The figure shows three views and two pictorial views of one solid part (mm, origin at its lowest corner). Answer the questions. Round coordinates to 2 decimals unless told otherwise and drop trailing zeros. Order: outer loops, then holes, each group sorted by start corner. A loop starts at its lowest first (then second) coordinate and runs counter-clockwise, first axis right, second up. Notation, with made-up numbers: M 4.5,58 L 35.5,58 A15 cw 35.5,75 Z; hole C -29,2.25 d10. An arc over 180 degrees is marked long. Return JSON: item names as keys, results as strings.
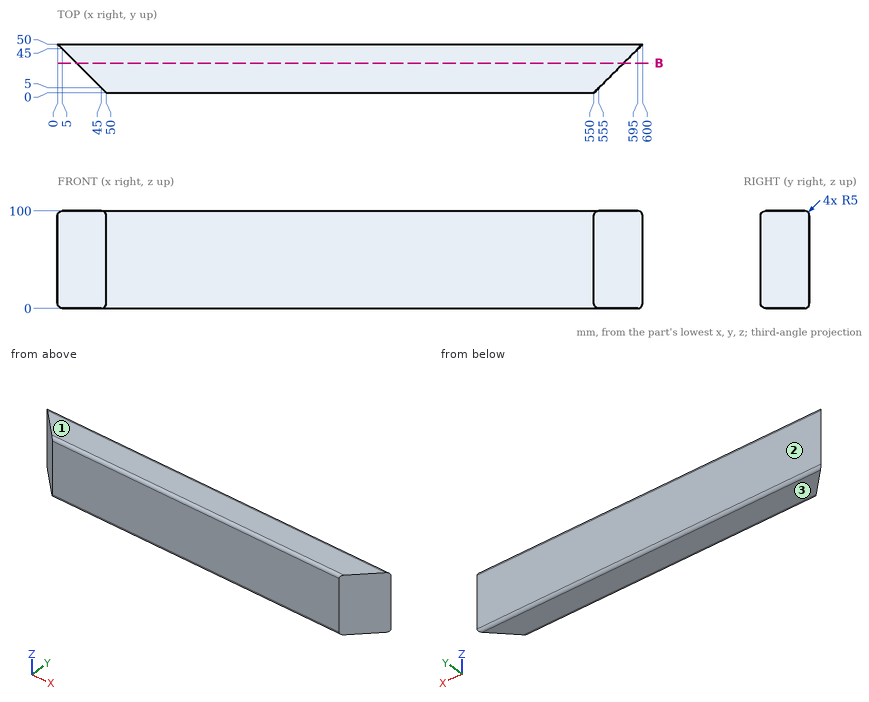
Item 1: Each of these flat-tipped pins is pushed along its axis until it touches: pin 1 (1 mm diameter, centred on y = 17.5, z = 34.5, fed in from +X); pin 2 (4 mm diameter, centred on y = 37, z = 43, fed in from -X); pin 3 (12 mm diameter, centred on y = 24.5, z = 48.5, fed in from -X). Where does it stop, or does it pass through?
Output:
{"pin 1": "stops at x = 568", "pin 2": "stops at x = 11", "pin 3": "stops at x = 19.5"}
Item 2: The mould has two halves that part along Z. Classify the marked faces 1, 2 and 3: pulls with the +Z half, pulls with the -Z half, needs draft (parallel to the pull), parting line crosses it, or undercut.
Output:
{"face 1": "pulls with the +Z half", "face 2": "needs draft", "face 3": "pulls with the -Z half"}
Item 3: Find section B-B (y = 30.5). Determine the outline of the cut face in (x, z), plus the area to 3 significant figures.
Output:
{"outline": "M 19.5,0 L 580.5,0 L 580.5,100 L 19.5,100 Z", "area": "56,100 mm^2"}
Item 4: Consider line 1 along Z through (x, y) = (149, 4.5); line 2 along X through (y, z) = (14, 7); line 3 along X through (y, z) = (33.5, 52). Determine where each line is inside the solid, lowest interval first. Write a range as [from, to].
Output:
{"line 1": "z = [0.03, 99.97]", "line 2": "x = [36, 564]", "line 3": "x = [16.5, 583.5]"}
